Can you work these out from the model? Positions are in its coordinate system, mm. Round coordinates to 2 decimals unless told otherwise and drop trailing zeros. Order: outer loops, then holes, each group sorted by start corner. A loop starts at its lowest first (then second) coordinate and runs counter-clockwise, first axis right, second up. Notation, with made-up numbers: M -13,-38 L 34,-38 A17 ccw 34,-6 Z; hole C 32,74 d8. An arc over 180 degrees is marked long. Answer as a JSON object with one key per item and string values. Group by question number.
```python
from build123d import *

# Parameters (mm, degrees)
SKETCH1_R      = 3.048
EXTRUDE1_DEPTH = 38.1
CHAMFER1_SIZE  = 0.6096
EXTRUDE7_DEPTH = 26.4


with BuildPart() as part:
    # Sketch1 → Extrude1 (new body, symmetric)
    with BuildSketch(Plane.XY):
        Circle(SKETCH1_R)
    extrude(amount=EXTRUDE1_DEPTH, both=True)

    # Chamfer1
    chamfer1_edges = [part.edges().sort_by_distance(p)[0] for p in [
        (-3.048, 0, -38.1),
        (-3.048, 0, 38.1),
    ]]
    chamfer(chamfer1_edges, length=CHAMFER1_SIZE)

    # Sketch13 → Extrude7 (cut, through all)
    with BuildSketch(Plane.XY.offset(12.7)):
        with BuildLine():
            Line((-1.524, 2.639645431), (1.524, 2.639645431))
            ThreePointArc((1.524, 2.639645431), (0, 3.048), (-1.524, 2.639645431))
        make_face()
    extrude(amount=EXTRUDE7_DEPTH, mode=Mode.SUBTRACT)


solid = part.part
```
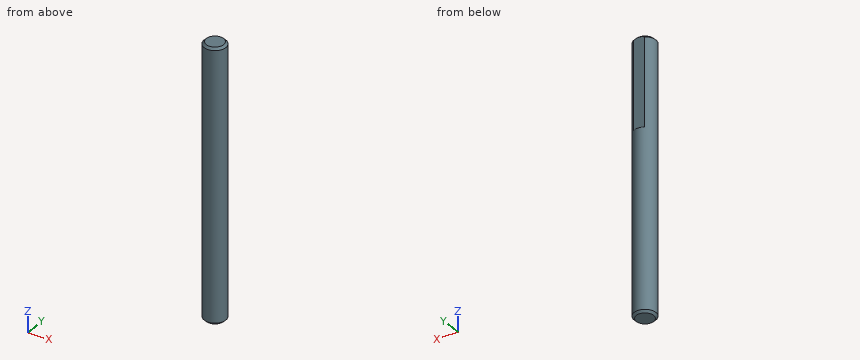
1) If we section it at B-B on z = -11: Write out the boundary of the cut face in (x, y), plus the area to 3 significant figures.
2) If we section it at C-C on z = 20.5: Write out the boundary of the cut face in (x, y), plus the area to 3 significant figures.
3) I need wall thicknesses on line 1 along Y through (x, z) = (-0.25, -32.5); line 2 along Y through (x, z) = (-2.5, -14.5); line 3 along X through (y, z) = (-0.75, -8). Which ranges of each line are inside material? Lowest first, please.
4) For pin 1 (3 mm diameter, centred on y = -1, z = 15, fed in from +X); pin 2 (3.5 mm diameter, centred on x = 0.5, z = 30, fed in from +Y); pin 3 (1.5 mm diameter, centred on x = 1, z = 20.5, fed in from -Y); pin 4 (1 mm diameter, centred on x = 1.5, z = -23, fed in from -Y), each with a flat end and sliding along its axis, tell me the tip position at first contact or that it passes through.
5) If we section it at A-A on x = 0: Write out the boundary of the cut face in (y, z), plus the area to 3 significant figures.
Findings:
{
 "1": {"outline": "C 0,0 d6.1", "area": "29.2 mm^2"},
 "2": {"outline": "M -1.52,2.64 A3.05 ccw long 1.52,2.64 Z", "area": "28.3 mm^2"},
 "3": {"line 1": "y = -3.04 to 3.04", "line 2": "y = -1.74 to 1.74", "line 3": "x = -2.95 to 2.95"},
 "4": {"pin 1": "stops at x = 3.05", "pin 2": "stops at y = 2.64", "pin 3": "stops at y = -3.04", "pin 4": "stops at y = -2.88"},
 "5": {"outline": "M -3.05,-37.49 L -2.44,-38.1 L 2.44,-38.1 L 3.05,-37.49 L 3.05,12.7 L 2.64,12.7 L 2.64,37.9 L 2.44,38.1 L -2.44,38.1 L -3.05,37.49 Z", "area": "454 mm^2"}
}
